Autodesk Inventor part; units mm, degrees
ref_plane "Start Plane" through (0, 0, 0) normal (0, 1, 0) x (-1, 0, 0)
ref_plane "End Plane" through (0, 304.8, 0) normal (0, 1, 0) x (-1, 0, 0)
ref_plane "YZ Plane" through (0, 0, 0) normal (1, 0, 0) x (0, 1, 0)
ref_plane "Start Plane" through (0, 0, 0) normal (0, 1, 0) x (-1, 0, 0)
ref_plane "End Plane" through (0, 304.8, 0) normal (0, 1, 0) x (-1, 0, 0)
sketch "Sketch" plane through (0, 0, 0) normal (0, 1, 0) x (-1, 0, 0)
  line L0 (8, -10) -> (-8, -10)
  line L1 (-10, -8) -> (-10, 8)
  line L2 (-8, 10) -> (8, 10)
  line L3 (10, 8) -> (10, -8)
  line L4 (10, -10) -> (-10, 10) construction
  line L5 (-10, -10) -> (10, 10) construction
  line L6 (14, -14) -> (-14, 14) construction
  line L7 (-14, -14) -> (14, 14) construction
  arc A0 (8, -10) -> (10, -8) centre (8, -8) ccw
  arc A1 (-10, -8) -> (-8, -10) centre (-8, -8) ccw
  arc A2 (-8, 10) -> (-10, 8) centre (-8, 8) ccw
  arc A3 (10, 8) -> (8, 10) centre (8, 8) ccw
  arc A4 (8, -14) -> (14, -8) centre (8, -8) ccw
  arc A5 (-14, -8) -> (-8, -14) centre (-8, -8) ccw
  arc A6 (-8, 14) -> (-14, 8) centre (-8, 8) ccw
  arc A7 (14, 8) -> (8, 14) centre (8, 8) ccw
  line L8 (3, -14) -> (3, -12)
  line L9 (3, -12) -> (-3, -12)
  line L10 (-3, -12) -> (-3, -14)
  line L11 (-14, -3) -> (-12, -3)
  line L12 (-12, -3) -> (-12, 3)
  line L13 (-12, 3) -> (-14, 3)
  line L14 (-3, 14) -> (-3, 12)
  line L15 (-3, 12) -> (3, 12)
  line L16 (3, 12) -> (3, 14)
  line L17 (14, 3) -> (12, 3)
  line L18 (12, 3) -> (12, -3)
  line L19 (12, -3) -> (14, -3)
  line L20 (0, -10) -> (0, -12) construction
  line L21 (-10, 0) -> (-12, 0) construction
  line L22 (0, 10) -> (0, 12) construction
  line L23 (10, 0) -> (12, 0) construction
  line L24 (14, 8) -> (14, 3)
  line L25 (14, -3) -> (14, -8)
  line L26 (8, -14) -> (3, -14)
  line L27 (-3, -14) -> (-8, -14)
  line L28 (-14, -8) -> (-14, -3)
  line L29 (-14, 3) -> (-14, 8)
  line L30 (-8, 14) -> (-3, 14)
  line L31 (3, 14) -> (8, 14)
  point P0 (0, 0)
  dimension "d1" = 20
  dimension "d2" = 2
  dimension "d3" = 6
  dimension "d4" = 20
  dimension "d5" = 6
  dimension "d6" = 2
  dimension "d8" = 28
extrude "Body" add sketch "Sketch" along normal up to surface (304.8 mm away) from surface at 0
sketch "Sketch2" plane through (0, 0, 0) normal (0, 1, 0) x (-1, 0, 0)
  line L0 (0, 0) -> (10, 0)
ref_plane "Work Plane3" through (0, 0, 0) normal (0, 0, -1) x (-1, 0, 0)
sketch "Sketch3" plane through (0, 0, 0) normal (0, 0, -1) x (-1, 0, 0)
  line L0 (-2, 0) -> (12, 0) construction
  line L1 (-2, 304.8) -> (12, 304.8) construction
  dimension "d16" = 304.8
equation "\"G_OFFSET_START\" = 0"
equation "\"G_OFFSET_END\" = 0"
equation "\"d12\" = Length + G_OFFSET_END"
equation "\"G_L\" = d16"
properties part number "CE-5.2.2-PR" material "Steel, Mild"
Geometry: final body of the model. Coordinates: model frame, mm. A direction names the side the tool comes from. Round coordinates to 2 decimals unless told otherwise and drop trailing zeros. Write each loop counter-clockwise with the first axis right and the second up, starting at its lowest first coordinate (ties: lowest second). Pieces come first, ordered by that corner, then holes. Notation, with made-up numbers: M 70.25,10.25 L 83.25,10.25 A15 ccw 83.25,17.25 Z; hole C 7.5,14 d4. An arc over 180 degrees is marked long. Answer in a Markdown table with one row per item. Add a question column.
(1) Cut plane B-B, the plane x = 5.5. Return the cut outline in (y, z), then the cut area to 3 significant figures.
(2) Contact query for flat-ended pins moving along their axis: pin 1 (1 mm diameter, centred on y = 172, z = 13, fed in from +X); pin 2 (0.6 mm diameter, centred on x = 13, y = 224.5, fed in from -Z); pin 3 (1.6 mm diameter, centred on x = -13, y = 92, fed in from -Z). Output: stop coordinate, or through.
(3) Reachability of faces 1 (the face through (-12.196, 150.266, 12.289)), 2 (the face through (-10, 150, 0)), 3 (the face through (-12, 150, 0)), 4 (the face through (12, 150, 0)), 5 (the face through (0, 150, -12)) from +Z, -Z, +X, -X, +Y, -Y: full face, straight path, thin tool, end or side. Return the list, or none.
(4) Ray query, L1, parallel to X at y = 106, z = 0.5; L2, parallel to Z at x = 3.5, y = 196. Return the intervals inside material, ascending.
Established:
| question | item | result |
|---|---|---|
| 1 | outline | M 0,-14 L 304.8,-14 L 304.8,-10 L 0,-10 Z; M 0,10 L 304.8,10 L 304.8,14 L 0,14 Z |
| 1 | area | 2,440 mm² |
| 2 | pin 1 | x = 11.97 |
| 2 | pin 2 | z = -11.73 |
| 2 | pin 3 | z = -12.28 |
| 3 | face 1 | +Z, -X, +Y, -Y |
| 3 | face 2 | +Y, -Y |
| 3 | face 3 | -X, +Y, -Y |
| 3 | face 4 | +X, +Y, -Y |
| 3 | face 5 | -Z, +Y, -Y |
| 4 | L1 | -12 to -10, 10 to 12 |
| 4 | L2 | -14 to -10, 10 to 14 |
